from build123d import *

# Parameters (mm, degrees)
SKETCH1_R           = 2.794
SKETCH1_W           = 7.62
SKETCH1_H           = 5.08
BOSS_EXTRUDE1_DEPTH = 1.905
FILLET1_R           = 1.27


with BuildPart() as part:
    # Sketch1 → Boss-Extrude1 (new, symmetric)
    with BuildSketch(Plane.XY):
        with BuildLine():
            Line((3.360104165, 3.81), (18.288, 3.81))
            Line((18.288, 3.81), (18.288, -3.81))
            Line((18.288, -3.81), (3.360104165, -3.81))
            ThreePointArc((3.360104165, -3.81), (-5.08, 0), (3.360104165, 3.81))
        make_face()
        with Locations(Location((0, 0, 0), (0, 0, 180))):
            Circle(SKETCH1_R, mode=Mode.SUBTRACT)
        with Locations((13.208, 0)):
            Rectangle(SKETCH1_W, SKETCH1_H, mode=Mode.SUBTRACT)
    extrude(amount=BOSS_EXTRUDE1_DEPTH, both=True)

    # Fillet1
    fillet1_edges = [part.edges().sort_by_distance(p)[0] for p in [
        (3.360104165, 3.81, 0),
        (18.288, 3.81, 0),
        (18.288, -3.81, 0),
        (3.360104165, -3.81, 0),
    ]]
    fillet(fillet1_edges, radius=FILLET1_R)


solid = part.part
Geometry: final body of the model. Coordinates: model frame, mm. A direction names the side the tool comes from. Round coordinates to 2 decimals unless told otherwise and drop trailing zeros. Loops run counter-clockwise (first coordinate to the right, second up) from the corner with the lowest first, then second, coordinate; pieces in that order, holes last. Notation, with made-up numbers: (42, -36.5) -> (94, -36.5) arc R27 cw to (94, -7.5) -> close; hole circle Ø3 at (-10.75, 6.5). An arc over 180 degrees is marked (long way). One line per question, with ' | ' between items. Start each with the question number.
1. Section D-D on x = 0. Output: boundary loops of the cut face in (y, z) (3 decimals).
2. Section B-B on y = 0. Output: boundary loops of the cut face in (x, z) (3 decimals).
3. Section A-A on x = 11.5. Output: boundary loops of the cut face in (y, z) (3 decimals), and give its area (3 significant figures).
4. Contact query for flat-ended pins moving along their axis: pin 1 (1 mm diameter, centred on x = 9.5, z = 0, fed in from -Y); pin 2 (1 mm diameter, centred on x = 8, z = 0.5, fed in from +Y). Output: stop coordinate, or through.
5. Section C-C on z = -0.1. Output: boundary loops of the cut face in (x, y), and give its area (3 significant figures).
6. Line query: line 1 along Y through (x, z) = (9.75, -0.3); line 2 along X through (y, z) = (1.75, 1.1); line 3 along Y through (x, z) = (0, -0.7). Output: solid intervals per line, ascending. Write a range as [from, to].
7. Set-up query: faces 4 (the face through (13, -2.54, 0)), 5 (the face through (11, -3.81, 0)), 6 (the face through (7, 0, -1.905)). Return all of +Z, -Z, +X, -X, +Y, -Y with unobstructed straight access to the full face (end or side cutting, diameter ignored); none if empty.
8. Mould query, pull axis Y, two halves, no side actions, for faces 1 (the face through (-5.078, -0.157, 0.027)), 2 (the face through (10, 3.81, 0)), 3 (the face through (13, 2.54, 0)). Classes: pulls with the +Y half, pulls with the -Y half, needs draft (parallel to the pull), parting line crosses it, or undercut.
Returned:
1) outline: (-5.08, -1.905) -> (-2.794, -1.905) -> (-2.794, 1.905) -> (-5.08, 1.905) -> close; (2.794, -1.905) -> (5.08, -1.905) -> (5.08, 1.905) -> (2.794, 1.905) -> close
2) outline: (-5.08, -1.905) -> (-2.794, -1.905) -> (-2.794, 1.905) -> (-5.08, 1.905) -> close; (2.794, -1.905) -> (9.398, -1.905) -> (9.398, 1.905) -> (2.794, 1.905) -> close; (17.018, -1.905) -> (18.288, -1.905) -> (18.288, 1.905) -> (17.018, 1.905) -> close
3) outline: (-3.81, -1.905) -> (-2.54, -1.905) -> (-2.54, 1.905) -> (-3.81, 1.905) -> close; (2.54, -1.905) -> (3.81, -1.905) -> (3.81, 1.905) -> (2.54, 1.905) -> close | area: 9.68 mm2
4) pin 1: stops at y = -3.81 | pin 2: stops at y = 3.81
5) outline: (3.05, -4.06) arc R1.27 cw to (3.81, -3.81) -> (17.02, -3.81) arc R1.27 ccw to (18.29, -2.54) -> (18.29, 2.54) arc R1.27 ccw to (17.02, 3.81) -> (3.81, 3.81) arc R1.27 cw to (3.05, 4.06) arc R5.08 ccw (long way) to start; hole circle Ø5.59 at (0, 0); hole (9.4, -2.54) -> (17.02, -2.54) -> (17.02, 2.54) -> (9.4, 2.54) -> close | area: 122 mm2
6) line 1: y = [-3.81, -2.54], [2.54, 3.81] | line 2: x = [-4.77, -2.18], [2.18, 9.4], [17.02, 18.29] | line 3: y = [-5.08, -2.79], [2.79, 5.08]
7) face 4: +Z, -Z | face 5: +Z, -Z, +X, -Y | face 6: -Z, +X, -X, +Y, -Y
8) face 1: parting line crosses it | face 2: pulls with the +Y half | face 3: undercut
